Geometry: final body of the model. Coordinates: model frame, mm. Face numbers are marked on the shaded views. A direction names the side the tool comes from. Round coordinates to 2 decimals unless told otherwise and drop trailing zeros. Loops run counter-clockwise (first coordinate to the right, second up) from the corner with the lowest first, then second, coordinate; pieces in that order, holes last. Notation, with made-up numbers: (66, 37) - (79, 37) arc R20 ccw to (79, 69) - close; hole circle Ø7 at (-3.5, -40). An arc over 180 degrees is marked (long way). Answer as a JSON object with one key per item and string values. Group by question number.
Item 1: Reachability of the marked faces 1 and 2 from +Z, -Z, +X, -X, +Y, -Y: full face, straight path, thin tool, end or side. Return the list, or none.
Item 2: Section D-D (x = -1). Return the cut outline in (y, z), plus the area to 3 significant figures.
Item 3: Section C-C (z = -18). Return the cut outline in (x, y), plus the area to 3 significant figures.
Item 4: Section A-A (y = 19.2). Return the cut outline in (x, z).
Item 5: Line query: line 1 (Y direction, x = -9.25, z = -10); line 2 (Z direction, x = 1.25, y = 5.75); line 3 (X direction, y = 14.25, z = -3.5). Output: solid intervals per line, ascending.
Item 6: First-contact query: pin 1 (6 mm diameter, centred on x = -3, y = 13, fed in from +Z); pin 2 (10 mm diameter, centred on y = 4, z = -16.5, fed in from -X); pin 3 (1.2 mm diameter, centred on y = 8.5, z = -13, fed in from -X). Flat tips, straight axial feed; report the tip coordinate or a pass-through.
Item 7: Section B-B (z = -10). Return the cut outline in (x, y).
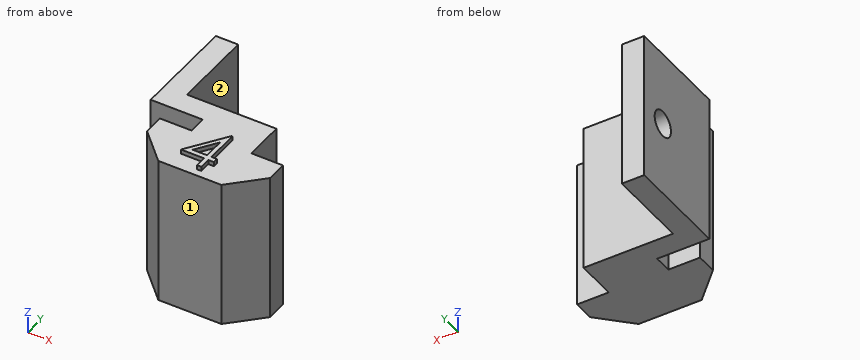
```python
from build123d import *

# Parameters (mm, degrees)
ESTRUSIONE_ESTRUSIONE1_DEPTH = 20
TAGLIO_ESTRUSIONE1_REACH     = 38.177
SCHIZZO6_R                   = 1.75
ESTRUSIONE_ESTRUSIONE2_DEPTH = 0.6


with BuildPart() as part:
    # Schizzo2 → Estrusione-Estrusione1 (new body)
    with BuildSketch(Plane.XY):
        Polygon((-4, 9.2), (-11, 9.2), (-11, 23.2), (-8, 23.2), (-8, 12.2), (4, 12.2), (4, 9.2), (4, 6.8), (8.25, 6.8), (8.25, 4.017766953), (4.232233047, 0), (-4.232233047, 0), (-8.25, 4.017766953), (-8.25, 6.8), (-4, 6.8), align=None)
    extrude(amount=-ESTRUSIONE_ESTRUSIONE1_DEPTH)

    # Schizzo6 → Taglio-Estrusione1 (cut, up to next)
    with BuildSketch(Plane.ZY.offset(11), mode=Mode.PRIVATE) as taglio_estrusione1_sk1:
        with Locations((-10, 19.2)):
            Circle(SCHIZZO6_R)
    taglio_estrusione1_tool1 = extrude(taglio_estrusione1_sk1.sketch, amount=-TAGLIO_ESTRUSIONE1_REACH, mode=Mode.PRIVATE) & part.part
    add(taglio_estrusione1_tool1.solids().sort_by_distance((-11, 19.2, -10))[0], mode=Mode.SUBTRACT)

    # Schizzo7 → Estrusione-Estrusione2 (add)
    with BuildSketch(Plane.XY):
        Polygon((0.798177083, 7.666666667), (0.916666667, 7.666666667), (0.916666667, 3.166666667), (1.666666667, 3.166666667), (1.666666667, 2.5), (0.916666667, 2.5), (0.916666667, 1), (0.333333333, 1), (0.333333333, 2.5), (-2.75, 2.5), align=None)
        Polygon((0.333333333, 3.166666667), (0.333333333, 5.989583333), (-1.604166667, 3.166666667), align=None, mode=Mode.SUBTRACT)
    extrude(amount=ESTRUSIONE_ESTRUSIONE2_DEPTH)


solid = part.part
```
Values:
{
 "1": {"face 1": "+Z, -Z, +X, -X, -Y", "face 2": "+Z, -Z, +X, +Y"},
 "2": {"outline": "(0, -20) - (12.2, -20) - (12.2, 0) - (5.05, 0) - (5.05, 0.6) - (4.05, 0.6) - (4.05, 0) - (3.17, 0) - (3.17, 0.6) - (2.5, 0.6) - (2.5, 0) - (0, 0) - close", "area": "245 mm^2"},
 "3": {"outline": "(-11, 9.2) - (-4, 9.2) - (-4, 6.8) - (-8.25, 6.8) - (-8.25, 4.02) - (-4.23, 0) - (4.23, 0) - (8.25, 4.02) - (8.25, 6.8) - (4, 6.8) - (4, 12.2) - (-8, 12.2) - (-8, 23.2) - (-11, 23.2) - close", "area": "193 mm^2"},
 "4": {"outline": "(-11, -20) - (-8, -20) - (-8, -11.75) - (-11, -11.75) - close; (-11, -8.25) - (-8, -8.25) - (-8, 0) - (-11, 0) - close"},
 "5": {"line 1": "y = 9.2 to 17.45, 20.95 to 23.2", "line 2": "z = -20 to 0", "line 3": "x = -11 to -8"},
 "6": {"pin 1": "stops at z = 0", "pin 2": "stops at x = -8.25", "pin 3": "stops at x = -4"},
 "7": {"outline": "(-11, 9.2) - (-4, 9.2) - (-4, 6.8) - (-8.25, 6.8) - (-8.25, 4.02) - (-4.23, 0) - (4.23, 0) - (8.25, 4.02) - (8.25, 6.8) - (4, 6.8) - (4, 12.2) - (-8, 12.2) - (-8, 17.45) - (-11, 17.45) - close; (-11, 20.95) - (-8, 20.95) - (-8, 23.2) - (-11, 23.2) - close"}
}
